Check sheet for the modelled part. Datum: model origin and axes. Units: mm. Face numbers are marked on the shaded views. A direction names the side the tool comes from. Round coordinates to 2 decimals unless told otherwise and drop trailing zeros. Write each loop counter-clockwise with the first axis right and the second up, starting at its lowest first coordinate (ties: lowest second). Pieces come first, ordered by that corner, then holes. Notation, with made-up numbers: M 41.25,84 L 73.25,84 A19 ccw 73.25,116 Z; hole C 47.5,45.5 d6. An arc over 180 degrees is marked long. Answer in a Markdown table with one row per item.
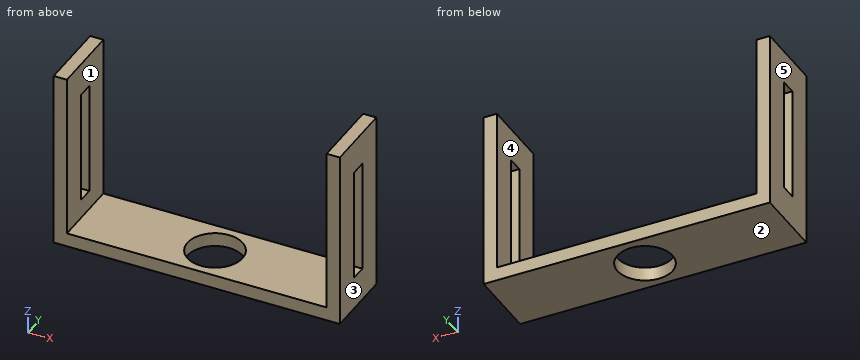
```python
from build123d import *

# Parameters (mm, degrees)
SKETCH1_W           = 52
SKETCH1_H           = 13
BOSS_EXTRUDE1_DEPTH = 2.5
SKETCH2_W           = 2.4
SKETCH2_H           = 13
BOSS_EXTRUDE2_DEPTH = 30
SKETCH3_W           = 20.5
SKETCH3_H           = 3
CUT_EXTRUDE1_DEPTH  = 55
SKETCH4_R           = 5
CUT_EXTRUDE2_DEPTH  = 55


with BuildPart() as part:
    # Sketch1 → Boss-Extrude1 (new body)
    with BuildSketch(Plane.XY):
        with Locations((26, -6.5)):
            Rectangle(SKETCH1_W, SKETCH1_H)
    extrude(amount=BOSS_EXTRUDE1_DEPTH)

    # Sketch2 → Boss-Extrude2 (add)
    with BuildSketch(Plane.XY.offset(2.5)):
        with Locations((1.2, -6.5)):
            Rectangle(SKETCH2_W, SKETCH2_H)
        with Locations((50.8, -6.5)):
            Rectangle(SKETCH2_W, SKETCH2_H)
    extrude(amount=BOSS_EXTRUDE2_DEPTH)

    # Sketch3 → Cut-Extrude1 (cut)
    with BuildSketch(Plane.ZY):
        with Locations((16.25, -6.5)):
            Rectangle(SKETCH3_W, SKETCH3_H)
    extrude(amount=-CUT_EXTRUDE1_DEPTH, mode=Mode.SUBTRACT)

    # Sketch4 → Cut-Extrude2 (cut)
    with BuildSketch(Plane.XY.offset(2.5)):
        with Locations((26, -6.5)):
            Circle(SKETCH4_R)
    extrude(amount=-CUT_EXTRUDE2_DEPTH, mode=Mode.SUBTRACT)


solid = part.part
```
1. Section check C-C, the plane x = 26. Record the cut outline in (y, z).
Found:
| item | result |
|---|---|
| outline | M -13,0 L -11.5,0 L -11.5,2.5 L -13,2.5 Z; M -1.5,0 L 0,0 L 0,2.5 L -1.5,2.5 Z |
2. Section check A-A, the plane z = 9.5. Record the cut outline in (x, y).
Found:
| item | result |
|---|---|
| outline | M 0,-13 L 2.4,-13 L 2.4,-8 L 0,-8 Z; M 0,-5 L 2.4,-5 L 2.4,0 L 0,0 Z; M 49.6,-13 L 52,-13 L 52,-8 L 49.6,-8 Z; M 49.6,-5 L 52,-5 L 52,0 L 49.6,0 Z |
3. Section check D-D, the plane y = -3.5. Record the cut outline in (x, z), and give its area (3 significant figures).
Found:
| item | result |
|---|---|
| outline | M 0,0 L 22,0 L 22,2.5 L 2.4,2.5 L 2.4,32.5 L 0,32.5 Z; M 30,0 L 52,0 L 52,32.5 L 49.6,32.5 L 49.6,2.5 L 30,2.5 Z |
| area | 254 mm2 |
4. Scan lines: L1, parallel to X at y = -8, z = 28.5; L2, parallel to Y at x = 26, z = 1; L3, parallel to Z at x = 35, y = -9.25. Record each from-to range of solid material in increasing order.
Found:
| item | result |
|---|---|
| L1 | x = 0 to 2.4, 49.6 to 52 |
| L2 | y = -13 to -11.5, -1.5 to 0 |
| L3 | z = 0 to 2.5 |
5. Draft check along X on the marked faces 3, 4 and 5. Enter one of: +X half, -X half, draft (parallel to the pull), parting line (faces both ways), or undercut.
Found:
| item | result |
|---|---|
| face 3 | +X half |
| face 4 | undercut |
| face 5 | -X half |
6. Section check B-B, the plane y = -6.5. Record the cut outline in (x, z).
Found:
| item | result |
|---|---|
| outline | M 0,0 L 21,0 L 21,2.5 L 2.4,2.5 L 2.4,6 L 0,6 Z; M 0,26.5 L 2.4,26.5 L 2.4,32.5 L 0,32.5 Z; M 31,0 L 52,0 L 52,6 L 49.6,6 L 49.6,2.5 L 31,2.5 Z; M 49.6,26.5 L 52,26.5 L 52,32.5 L 49.6,32.5 Z |
7. Access from +Z, -Z, +X, -X, +Y, -Y to the whole of each face (thin tool, end or side, straight path). Record for the marked faces 1 and 2.
Found:
| item | result |
|---|---|
| face 1 | +Z, +Y, -Y |
| face 2 | -Z, +X, -X, +Y, -Y |
